CAD build for the part. Positions are in the model's coordinates, mm. A direction names the side the tool comes from. Coordinates: 2 decimals unless noted, no trailing zeros. Order: outer loops, then holes, each group sorted by start corner. A loop starts at its lowest first (then second) coordinate and runs counter-clockwise, first axis right, second up. Notation, with made-up numbers: M -31,31 L -8,31 A12 cw -8,35 Z; hole C 60,-15.75 d6. An arc over 180 degrees is marked long. One line per item, written item: value.
Autodesk Inventor part; units mm, degrees
ref_plane "YZ Plane" through (0, 0, 0) normal (1, 0, 0) x (0, 1, 0)
ref_plane "XZ Plane" through (0, 0, 0) normal (0, 1, 0) x (-1, 0, 0)
ref_plane "XY Plane" through (0, 0, 0) normal (0, 0, 1) x (1, 0, 0)
sketch "Sketch1" plane through (0, 0, 0) normal (1, 0, 0) x (0, 1, 0)
  line L0 (0, 0) -> (0, -24.25)
  line L1 (0, 0) -> (0, 24.25)
  line L2 (0, 0) -> (33.993, 0)
  circle A0 centre (33.993, 0) radius 51.7565
  circle A1 centre (33.993, 0) radius 43.8815
  dimension "d0" = 24.25
  dimension "d1" = 24.25
  dimension "d2" = 33.993
  dimension "d3" = 103.513
  dimension "d17" = 87.763
extrude "Extrusion1" add sketch "Sketch1" along normal blind 9.271
sketch "Sketch5" plane through (0, 33.993, 0) normal (-1, 0, 0) x (0, 0, 1)
  circle A0 centre (0, 0) radius 43.8815
  point P0 (0, -33.993)
extrude "Extrusion5" add sketch "Sketch5" against normal blind 4.271
sketch "Sketch6" plane through (4.271, 33.993, 0) normal (1, 0, 0) x (0, 0, -1)
  line L0 (0, 0) -> (17.056, 0)
  line L1 (0, 0) -> (-17.056, 0)
  circle A0 centre (-17.056, 0) radius 2.5
  circle A1 centre (17.056, 0) radius 2.5
  circle A2 centre (0, 0) radius 6.25
  line L2 (-17.056, 0) -> (-17.056, -15)
  line L3 (-17.056, 0) -> (-17.056, 15)
  line L4 (17.056, 0) -> (17.056, 15)
  line L5 (17.056, 0) -> (17.056, -15)
  circle A3 centre (-17.056, 15) radius 2.5
  circle A4 centre (-17.056, -15) radius 2.5
  circle A5 centre (17.056, 15) radius 2.5
  circle A6 centre (17.056, -15) radius 2.5
  point P0 (0, -33.993)
  dimension "d22" = 17.056
  dimension "d23" = 17.056
  dimension "d24" = 5
  dimension "d25" = 5
  dimension "d26" = 12.5
  dimension "d29" = 15
  dimension "d30" = 15
  dimension "d31" = 15
  dimension "d32" = 15
  dimension "d33" = 5
  dimension "d34" = 5
  dimension "d35" = 5
  dimension "d36" = 5
extrude "Extrusion6" cut sketch "Sketch6" against normal blind 4.271
properties part number "4ax_plate_joint"
Q1. Which spindle directions (+Z, -Z, +X, -X, +Y, -Y) get a long thin tool onto all of the face, cutting with end or side? Do faces 4 (the face through (6.74, -0.83, 26.7)), 5 (the face through (2.2, 27.9, 1.4)). Say none if no direction does.
Recorded:
face 4: +X
face 5: +X, -X
Q2. Slice it at B-B (y = 39). List the corners of the cut face in (x, z).
Recorded:
outline: M 0,-51.51 L 9.27,-51.51 L 9.27,-43.59 L 4.27,-43.59 L 4.27,-3.74 L 0,-3.74 Z; M 0,3.74 L 4.27,3.74 L 4.27,43.59 L 9.27,43.59 L 9.27,51.51 L 0,51.51 Z
Q3. Slice it at D-D (z = 28.5). List the corners of the cut face in (x, y).
Recorded:
outline: M 0,-9.21 L 9.27,-9.21 L 9.27,0.63 L 4.27,0.63 L 4.27,67.36 L 9.27,67.36 L 9.27,77.2 L 0,77.2 Z
Q4. Pin check, flat tips, straight feed: pin 1 Ø1 at (x, z) = (3, 24) entering from +Y; pin 2 Ø4 at (y, z) = (52, 4) entering from +X; pin 3 Ø4 at (y, z) = (48.993, 17.056) entering from +X; pin 4 Ø3 at (x, y) = (7.5, 49.5) entering from -Z. Stop position of each tip, or through.
Recorded:
pin 1: stops at y = 80.11
pin 2: stops at x = 4.27
pin 3: passes through
pin 4: stops at z = -49.83
Q5. Drill centre lines: line 1 along X through (y, z) = (26, -9); line 2 along Y through (x, z) = (7, 35); line 3 along Z through (x, y) = (3.75, 50). Where is each one in solid material? Low to high.
Recorded:
line 1: x = 0 to 4.27
line 2: y = -4.13 to 7.52, 60.46 to 72.12
line 3: z = -49.22 to -19.34, -14.77 to 14.77, 19.34 to 49.22
Q6. Slice it at A-A (z = 0). List the corners of the cut face in (x, y).
Recorded:
outline: M 0,-17.76 L 9.27,-17.76 L 9.27,-9.89 L 4.27,-9.89 L 4.27,27.74 L 0,27.74 Z; M 0,40.24 L 4.27,40.24 L 4.27,77.87 L 9.27,77.87 L 9.27,85.75 L 0,85.75 Z
Q7. Mould opens along Z. For faces 1 (the face through (4.271, 25, -1)), 2 (the face through (4.571, 81.803, 19.823)), 3 (the face through (0, 45, 1)) say: released by +Z, released by -Z, zero draft, split by the parting line, or undercut.
Recorded:
face 1: undercut
face 2: split by the parting line
face 3: zero draft
Q8. Slice it at C-C (x = 6.5). List the corners of the cut face in (y, z), plus the area to 3 significant figures.
Recorded:
outline: C 33.99,0 d103.51; hole C 33.99,0 d87.76
area: 2,370 mm^2
